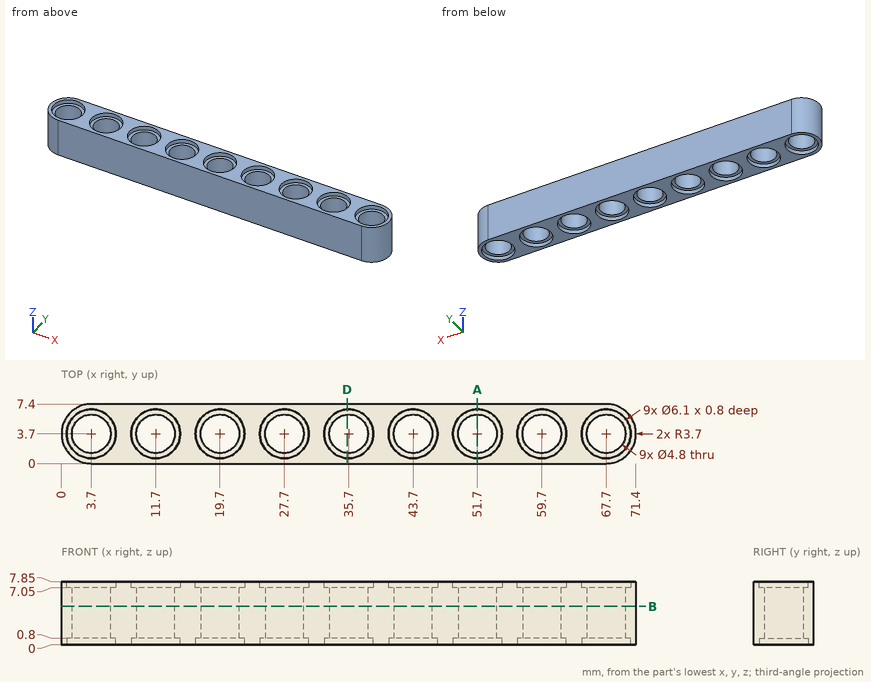
Study the drawing (mm; zero at the part's minimum x, y, z) and answer. Coordinates: 2 decimals unless noted, no trailing zeros. Write each loop counter-clockwise with the first axis right and the second up, starting at its lowest first coordinate (ties: lowest second). Pieces come first, ordered by that corner, then holes. Notation, with made-up numbers: (26, -5) - (56, -5) arc R7 cw to (56, 5) - close; hole circle Ø8 at (3, 13.5). An arc over 180 degrees is marked (long way). Return JSON: item names as keys, results as strings. Group by question number.
1. A cutting plane is placed at D-D, the plane x = 35.5. Determine the outline of the cut face in (y, z).
2. Given pin 1 (3.5 mm diameter, centred on x = 43.7, y = 3.7, fed in from +Z); pin 2 (2 mm diameter, centred on y = 5.5, z = 2.5, fed in from -X); pin 3 (2 mm diameter, centred on x = 58.5, y = 4.5, fed in from -Z); pin 4 (4 mm diameter, centred on x = 13, y = 3.5, fed in from -Z), each flat-ended and moving along its own axis, determine where each tip first touches the part or whether it passes through.
3. A cutting plane is placed at B-B, the plane z = 4.75. Give the number of separate pieces and of enclosed holes in the cut face, plus the area to 3 significant figures.
4. Straight lines are drawn through the part: L1, parallel to Y at x = 27.7, z = 7.55; L2, parallel to Y at x = 11.7, z = 2.75; L3, parallel to Z at x = 59.5, y = 0.75. For each, find the intervals that lie inside material, in ascending order.
5. A cutting plane is placed at A-A, the plane x = 51.7. Determine the outline of the cut face in (y, z), plus the area to 3 significant figures.
Ans:
{
 "1": {"outline": "(0, 0) - (0.66, 0) - (0.66, 0.8) - (1.31, 0.8) - (1.31, 7.05) - (0.66, 7.05) - (0.66, 7.85) - (0, 7.85) - close; (6.09, 0.8) - (6.74, 0.8) - (6.74, 0) - (7.4, 0) - (7.4, 7.85) - (6.74, 7.85) - (6.74, 7.05) - (6.09, 7.05) - close"},
 "2": {"pin 1": "through", "pin 2": "x = 0.09", "pin 3": "z = 0.8", "pin 4": "z = 0"},
 "3": {"separate pieces": "1", "enclosed holes": "9", "area": "354 mm²"},
 "4": {"L1": "0 to 0.65, 6.75 to 7.4", "L2": "0 to 1.3, 6.1 to 7.4", "L3": "0.8 to 7.05"},
 "5": {"outline": "(0, 0) - (0.65, 0) - (0.65, 0.8) - (1.3, 0.8) - (1.3, 7.05) - (0.65, 7.05) - (0.65, 7.85) - (0, 7.85) - close; (6.1, 0.8) - (6.75, 0.8) - (6.75, 0) - (7.4, 0) - (7.4, 7.85) - (6.75, 7.85) - (6.75, 7.05) - (6.1, 7.05) - close", "area": "18.3 mm²"}
}
